For this review, take the finished solid that the model builds, in its own axes (mm). Round coordinates to 2 decimals unless told otherwise and drop trailing zeros. Loops run counter-clockwise (first coordinate to the right, second up) from the corner with the lowest first, then second, coordinate; pieces in that order, holes last.
1. Draft analysis for pull direction Y (two halves, no side actions). For faces 1 (the cylindrical face through (18.97, -2.22, 50.85)), 2 (the flat face through (-9.48, 49.1, 14.83)), 3 (the flat face through (-9.48, -4.52, -30.17)), state which applies: released by +Y, released by -Y, zero draft, split by the parting line, or undercut.
2. Clearance check with flat-ended pins moving along their axes: pin 1 Ø3 at (y, z) = (13, 14) entering from +X; pin 2 Ø6.5 at (y, z) = (0, 52) entering from +X (3 decimals); pin 3 Ø8 at (x, y) = (11, 26) entering from -Z; pin 4 Ø4 at (y, z) = (3.5, 33.5) entering from -X. State where each tip first meets the part, or that it passes through.
3. To check wall thickness, follow line 1 along Y through (x, z) = (11.5, 22); line 2 along X through (y, z) = (0, 30) (3 decimals); line 3 along Y through (x, z) = (-14.5, 12.5). State the ranges of each line that lie inside material, in increasing order.
4. Consider section B-B on x = 0. State the section outline as (y, z) points (3 decimals), then the cut area to 3 significant figures.
5. Consider section C-C on x = -13.5. State the section outline as (y, z) points (3 decimals).
from build123d import *

# Parameters (mm, degrees)
SKETCH1_R               = 20.675
SKETCH1_R_2             = 17.5
BOSS_EXTRUDE1_DEPTH     = 60
SKETCH3_R               = 20.675
SKETCH3_R_2             = 10.5
BOSS_EXTRUDE2_DEPTH     = 70
BOSS_EXTRUDE5_REACH     = 44.266
SKETCH1_4_R             = 20.675
SKETCH1_4_R_2           = 17.5
SKETCH6_R               = 10.5
CUT_EXTRUDE1_DEPTH      = 37.812904316
CUT_EXTRUDE1_DEPTH_BACK = 91.360900294
SKETCH7_R               = 2.5
CUT_EXTRUDE2_DEPTH      = 21.675
CUT_EXTRUDE2_DEPTH_BACK = 21.675


with BuildPart() as part:
    # Sketch1 → Boss-Extrude1 (new body)
    with BuildSketch(Plane.XY):
        Circle(SKETCH1_R)
        Circle(SKETCH1_R_2, mode=Mode.SUBTRACT)
    extrude(amount=BOSS_EXTRUDE1_DEPTH)

    # Sketch3 → Boss-Extrude2 (add)
    with BuildSketch(Plane(origin=(0, 45.962666587, 18.567256581), x_dir=(1, 0, 0), z_dir=(0, 0.766044443, 0.64278761))):
        Circle(SKETCH3_R)
        Circle(SKETCH3_R_2, mode=Mode.SUBTRACT)
    extrude(amount=-BOSS_EXTRUDE2_DEPTH)

    # Sketch1<4> → Boss-Extrude5 (add, up to next)
    with BuildSketch(Plane.XY, mode=Mode.PRIVATE) as boss_extrude5_sk1:
        Circle(SKETCH1_4_R)
        Circle(SKETCH1_4_R_2, mode=Mode.SUBTRACT)
    boss_extrude5_tool1 = extrude(boss_extrude5_sk1.sketch, amount=-BOSS_EXTRUDE5_REACH, mode=Mode.PRIVATE) - part.part
    add(boss_extrude5_tool1.solids().sort_by_distance((-20.090223, 0, 0))[0])

    # Sketch6 → Cut-Extrude1 (cut, two sides)
    with BuildSketch(Plane(origin=(0, 36.114589057, 30.303738358), x_dir=(1, 0, 0), z_dir=(0, 0.766044443, 0.64278761))) as cut_extrude1_sk:
        with Locations((0, 15.320888862)):
            Circle(SKETCH6_R)
    extrude(amount=CUT_EXTRUDE1_DEPTH, mode=Mode.SUBTRACT)
    extrude(cut_extrude1_sk.sketch, amount=-CUT_EXTRUDE1_DEPTH_BACK, mode=Mode.SUBTRACT)

    # Sketch7 → Cut-Extrude2 (cut, two sides)
    with BuildSketch(Plane(origin=(0, 0, 0), x_dir=(0, 0, -1), z_dir=(1, 0, 0))) as cut_extrude2_sk:
        with Locations((-52, 0)):
            Circle(SKETCH7_R)
    extrude(amount=CUT_EXTRUDE2_DEPTH, mode=Mode.SUBTRACT)
    extrude(cut_extrude2_sk.sketch, amount=-CUT_EXTRUDE2_DEPTH_BACK, mode=Mode.SUBTRACT)


solid = part.part
Resolved:
1. face 1: undercut
1. face 2: released by +Y
1. face 3: released by -Y
2. pin 1: stops at x = 17.18
2. pin 2: stops at x = 20.675
2. pin 3: stops at z = -25.41
2. pin 4: stops at x = -20.62
3. line 1: y = -17.18 to -13.19, 13.19 to 17.18, 23.32 to 43.08
3. line 2: x = -20.675 to -17.5, 17.5 to 20.675
3. line 3: y = -14.74 to -9.8, 9.8 to 14.74, 15.8 to 51.05
4. outline: (-20.95, -10.59) - (-14.41, -18.384) - (39.213, 26.611) - (32.673, 34.405) - (20.675, 24.338) - (20.675, 60) - (17.5, 60) - (17.5, 21.674) - (-17.5, -7.695) - (-17.5, 60) - (-20.675, 60) - (-20.675, -10.359) - close; (-0.911, -34.471) - (5.629, -42.266) - (59.252, 2.729) - (52.712, 10.524) - close
4. area: 1,760 mm2
5. outline: (-17.726, -14.432) - (2.405, -38.423) - (56.028, 6.572) - (35.897, 30.563) - (15.659, 13.581) - (15.659, 60) - (11.136, 60) - (11.136, 9.785) - (-11.136, -8.902) - (-11.136, 60) - (-15.659, 60) - (-15.659, -12.698) - close
